Check sheet for the modelled part. Datum: model origin and axes. Units: mm. A direction names the side the tool comes from. Give positions to 0.01 mm unless a question says otherwise; leave off trailing zeros. Loops run counter-clockwise (first coordinate to the right, second up) from the corner with the lowest first, then second, coordinate; pieces in that order, holes last. Notation, with made-up numbers: (55, 57) -> (113, 57) arc R31 ccw to (113, 95) -> close; hole circle Ø1 at (26.5, 59.5). An arc over 180 degrees is marked (long way). Write each question's results on one line, items separated by ' | '. Start each with the question number.
1. Cross-section at B-B on z = 12.5. Record the boundary of the cut face in (x, y).
2. Gauge pin test, flat ends, axial feed: pin 1 Ø5 at (y, z) = (-34, 13.5) entering from -X; pin 2 Ø5 at (y, z) = (-31, 18.5) entering from +X; pin 3 Ø0.7 at (x, z) = (11, 22.5) entering from -Y; pin 4 Ø5 at (y, z) = (-0.5, 19) entering from -X. Record the tip position at first contact, or that the pin passes through.
3. Cross-section at A-A on y = -28. Record the boundary of the cut face in (x, z), and give its area (4 significant figures).
4. Material ranges on L1, parallel to X at y = 0, z = 15; L2, parallel to X at y = -33, z = 9.25; L3, parallel to Y at x = 0, z = 15.25, recorded low to high. Write a range as from..to.
5. Cross-section at D-D on x = 0. Record the boundary of the cut face in (y, z).
6. Mould release check, pull along Z, two halves, no side actions. Record for faces 1 (the face through (0, -15, 0)), 2 (the face through (5, -34, 7)), 3 (the face through (-12.1, -15.3, 11.7)), 4 (the face through (7.4, -33.6, 19.1)): +Z half, -Z half, draft (parallel to the pull), parting line (faces both ways), or undercut.
7. Tool access check on faces 5 (the face through (7.1, -43.98, 18.71)), 6 (the face through (-6.5, -34, 11)), 7 (the face through (-7.6, -33.6, 18.9)). Record the directions out of +Z, -Z, +X, -X, +Y, -Y that give a thin tool (end or side, any length) a straight path to the whole face; none if there is none.
8. Cross-section at C-C on y = 0. Record the boundary of the cut face in (x, z).
from build123d import *

# Parameters (mm, degrees)
BOSS_EXTRUDE1_DEPTH = 23
FILLET1_R           = 10
SKETCH2_W           = 13
SKETCH2_H           = 13
CUT_EXTRUDE1_DEPTH  = 20
CHAMFER2_SIZE       = 3.5
CUT_EXTRUDE2_DEPTH  = 26
CHAMFER3_SIZE       = 1
FILLET2_R           = 5


with BuildPart() as part:
    # Sketch1 → Boss-Extrude1 (new body)
    with BuildSketch(Plane.XY):
        with BuildLine():
            Line((-11.5, -14.491376746), (-11.5, -44.491376746))
            Line((-11.5, -44.491376746), (11.5, -44.491376746))
            Line((11.5, -44.491376746), (11.5, -14.491376746))
            ThreePointArc((11.5, -14.491376746), (17.862669336, -4.814046549), (17.224619009, 6.75))
            ThreePointArc((17.224619009, 6.75), (14.31318663, 8.736071822), (11.401754251, 6.75))
            ThreePointArc((11.401754251, 6.75), (0, -13.25), (-11.401754251, 6.75))
            ThreePointArc((-11.401754251, 6.75), (-14.31318663, 8.736071822), (-17.224619009, 6.75))
            ThreePointArc((-17.224619009, 6.75), (-17.862669336, -4.814046549), (-11.5, -14.491376746))
        make_face()
    extrude(amount=BOSS_EXTRUDE1_DEPTH)

    # Fillet1
    fillet1_edges = [part.edges().sort_by_distance(p)[0] for p in [
        (-11.5, -14.491376746, 11.5),
        (11.5, -14.491376746, 11.5),
    ]]
    fillet(fillet1_edges, radius=FILLET1_R)

    # Sketch2 → Cut-Extrude1 (cut)
    with BuildSketch(Plane.XZ.offset(44.491376746)):
        with Locations((0, 11.5)):
            Rectangle(SKETCH2_W, SKETCH2_H)
    extrude(amount=-CUT_EXTRUDE1_DEPTH, mode=Mode.SUBTRACT)

    # Chamfer2
    chamfer2_edges = [part.edges().sort_by_distance(p)[0] for p in [
        (-6.5, -34.491376746, 5),
        (-6.5, -34.491376746, 18),
        (6.5, -34.491376746, 18),
        (6.5, -34.491376746, 5),
    ]]
    chamfer(chamfer2_edges, length=CHAMFER2_SIZE)

    # Sketch3 → Cut-Extrude2 (cut)
    with BuildSketch(Plane.XZ.offset(44.491376746)):
        Polygon((-11.5, 15), (-3.5, 23), (-11.5, 23), align=None)
        Polygon((3.5, 23), (11.5, 15), (11.5, 23), align=None)
        Polygon((11.5, 0), (11.5, 8), (3.5, 0), align=None)
        Polygon((-11.5, 0), (-3.5, 0), (-11.5, 8), align=None)
    extrude(amount=-CUT_EXTRUDE2_DEPTH, mode=Mode.SUBTRACT)

    # Chamfer3
    chamfer3_edges = [part.edges().sort_by_distance(p)[0] for p in [
        (7.5, -44.491376746, 4),
        (7.5, -44.491376746, 19),
        (-7.5, -44.491376746, 19),
        (0, -44.491376746, 5),
        (-6.5, -44.491376746, 11.5),
        (6.5, -44.491376746, 11.5),
        (0, -44.491376746, 18),
        (-4.75, -44.491376746, 6.75),
        (4.75, -44.491376746, 6.75),
        (4.75, -44.491376746, 16.25),
        (-4.75, -44.491376746, 16.25),
        (0, -44.491376746, 0),
        (0, -44.491376746, 23),
        (11.5, -44.491376746, 11.5),
        (-11.5, -44.491376746, 11.5),
        (-7.5, -44.491376746, 4),
    ]]
    chamfer(chamfer3_edges, length=CHAMFER3_SIZE)

    # Fillet2
    # the kernel refuses this fillet: 5 mm, written as the material it adds along each edge
    with BuildSketch(Plane(origin=(20.338834765, -18.491376746, 16.838834765), x_dir=(0, -1, 0), z_dir=(-0.7071067811865476, 0, -0.7071067811865476))) as fillet2_piece_1_section:
        with BuildLine():
            CenterArc((FILLET2_R, -FILLET2_R), FILLET2_R, 90, 90)
            Line((0, -FILLET2_R), (0, 0))
            Line((0, 0), (FILLET2_R, 0))
        make_face()
    fillet2_piece_1 = extrude(amount=36.313708499, mode=Mode.PRIVATE)
    fillet2_piece_1 = split(fillet2_piece_1, bisect_by=Plane(origin=(11.5, -19.775050917, 3.381146021), z_dir=(-1, 0, 0)), keep=Keep.TOP, mode=Mode.PRIVATE)
    fillet2_piece_1 = split(fillet2_piece_1, bisect_by=Plane(origin=(8.118853979, -19.775050917, 0), z_dir=(0, 0, 1)), keep=Keep.TOP, mode=Mode.PRIVATE)
    add(fillet2_piece_1)
    with BuildSketch(Plane(origin=(-5.338834765, -18.491376746, 31.838834765), x_dir=(0, -1, 0), z_dir=(0.7071067811865476, 0, -0.7071067811865476))) as fillet2_piece_2_section:
        with BuildLine():
            CenterArc((FILLET2_R, -FILLET2_R), FILLET2_R, 90, 90)
            Line((0, -FILLET2_R), (0, 0))
            Line((0, 0), (FILLET2_R, 0))
        make_face()
    fillet2_piece_2 = extrude(amount=36.313708499, mode=Mode.PRIVATE)
    fillet2_piece_2 = split(fillet2_piece_2, bisect_by=Plane(origin=(8.118853979, -19.775050917, 23), z_dir=(0, 0, -1)), keep=Keep.TOP, mode=Mode.PRIVATE)
    fillet2_piece_2 = split(fillet2_piece_2, bisect_by=Plane(origin=(11.5, -19.775050917, 19.618853979), z_dir=(-1, 0, 0)), keep=Keep.TOP, mode=Mode.PRIVATE)
    add(fillet2_piece_2)
    with BuildSketch(Plane(origin=(-20.338834765, -18.491376746, 6.161165235), x_dir=(0, -1, 0), z_dir=(0.7071067811865476, 0, 0.7071067811865476))) as fillet2_piece_3_section:
        with BuildLine():
            CenterArc((FILLET2_R, -FILLET2_R), FILLET2_R, 90, 90)
            Line((0, -FILLET2_R), (0, 0))
            Line((0, 0), (FILLET2_R, 0))
        make_face()
    fillet2_piece_3 = extrude(amount=36.313708499, mode=Mode.PRIVATE)
    fillet2_piece_3 = split(fillet2_piece_3, bisect_by=Plane(origin=(-8.118853979, -19.775050917, 23), z_dir=(0, 0, -1)), keep=Keep.TOP, mode=Mode.PRIVATE)
    fillet2_piece_3 = split(fillet2_piece_3, bisect_by=Plane(origin=(-11.5, -19.775050917, 19.618853979), z_dir=(1, 0, 0)), keep=Keep.TOP, mode=Mode.PRIVATE)
    add(fillet2_piece_3)
    with BuildSketch(Plane(origin=(5.338834765, -18.491376746, -8.838834765), x_dir=(0, -1, 0), z_dir=(-0.7071067811865476, 0, 0.7071067811865476))) as fillet2_piece_4_section:
        with BuildLine():
            CenterArc((FILLET2_R, -FILLET2_R), FILLET2_R, 90, 90)
            Line((0, -FILLET2_R), (0, 0))
            Line((0, 0), (FILLET2_R, 0))
        make_face()
    fillet2_piece_4 = extrude(amount=36.313708499, mode=Mode.PRIVATE)
    fillet2_piece_4 = split(fillet2_piece_4, bisect_by=Plane(origin=(-8.118853979, -19.775050917, 0), z_dir=(0, 0, 1)), keep=Keep.TOP, mode=Mode.PRIVATE)
    fillet2_piece_4 = split(fillet2_piece_4, bisect_by=Plane(origin=(-11.5, -19.775050917, 3.381146021), z_dir=(1, 0, 0)), keep=Keep.TOP, mode=Mode.PRIVATE)
    add(fillet2_piece_4)


solid = part.part
Geometry says:
1) outline: (-17.22, 6.75) arc R18.5 ccw to (-13.96, -12.14) arc R10 cw to (-11.5, -18.71) -> (-11.5, -43.49) -> (-10.5, -44.49) -> (-7.5, -44.49) -> (-6.5, -43.49) -> (-6.5, -24.49) -> (6.5, -24.49) -> (6.5, -43.49) -> (7.5, -44.49) -> (10.5, -44.49) -> (11.5, -43.49) -> (11.5, -18.71) arc R10 cw to (13.96, -12.14) arc R18.5 ccw to (17.22, 6.75) arc R3.13 ccw to (11.4, 6.75) arc R13.25 cw (long way) to (-11.4, 6.75) arc R3.13 ccw to start
2) pin 1: x = -11.5 | pin 2: x = 10.5 | pin 3: y = -18.51 | pin 4: x = -18.5
3) outline: (-11.5, 8) -> (-3.5, 0) -> (3.5, 0) -> (11.5, 8) -> (11.5, 15) -> (3.5, 23) -> (-3.5, 23) -> (-11.5, 15) -> close; hole (-6.5, 8.5) -> (-3, 5) -> (3, 5) -> (6.5, 8.5) -> (6.5, 14.5) -> (3, 18) -> (-3, 18) -> (-6.5, 14.5) -> close | area: 256.5 mm^2
4) L1: -18.5..-13.25, 13.25..18.5 | L2: -11.5..-6.5, 6.5..11.5 | L3: -24.49..-13.25
5) outline: (-44.49, 1) -> (-43.49, 0) -> (-13.25, 0) -> (-13.25, 23) -> (-43.49, 23) -> (-44.49, 22) -> (-44.49, 19) -> (-43.49, 18) -> (-24.49, 18) -> (-24.49, 5) -> (-43.49, 5) -> (-44.49, 4) -> close
6) face 1: -Z half | face 2: undercut | face 3: draft | face 4: +Z half
7) face 5: +Z, +X, -Y | face 6: -Y | face 7: +Z, -X, -Y
8) outline: (-18.5, 0) -> (-13.25, 0) -> (-13.25, 23) -> (-18.5, 23) -> close; (13.25, 0) -> (18.5, 0) -> (18.5, 23) -> (13.25, 23) -> close
